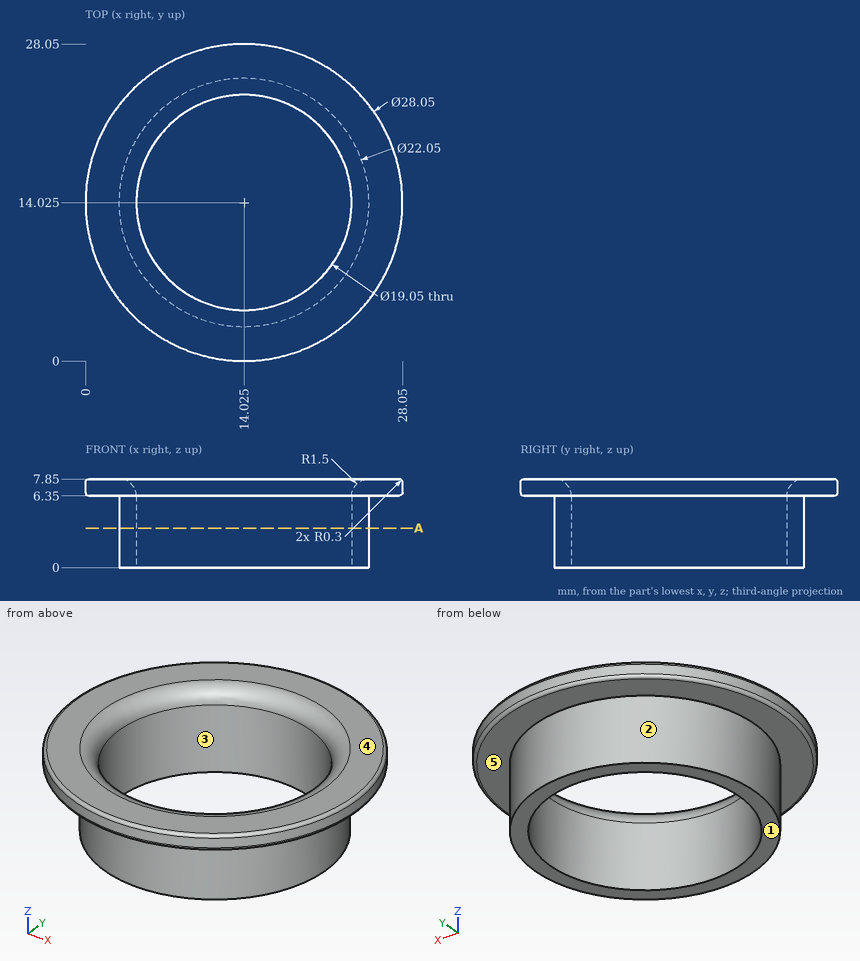
Could you check a few things on this drawing? It's one solid part, dimensions in mm from its lowest x, y, z. A direction names the side the tool comes from. Give positions to 0.01 mm unless a question says otherwise; leave off trailing zeros. Order: outer loops, then holes, each group sorted by start corner. A loop starts at its lowest first (then second) coordinate and runs counter-clockwise, first axis right, second up. Notation, with made-up numbers: M -16.75,-18 L -0.75,-18 A19 cw -0.75,14 Z; hole C -12.5,35 d10. An arc over 180 degrees is marked long. Use one line per item in the form item = value. Start each with the question number.
Item 1: Will these pins go through, and if not, where does the flat tip stop? pin 1 Ø1 at (y, z) = (12, 5.5) entering from -X; pin 2 Ø3 at (y, z) = (12, 4.5) entering from -X; pin 3 Ø2 at (x, z) = (12, 1.5) entering from -Y.
Item 2: If we section it at A-A (z = 3.5): Write out the boundary of the cut face in (x, y) (3 decimals), then the cut area to 3 significant figures.
Item 3: For the marked faces 4 and 5, which set-ups out of +Z, -Z, +X, -X, +Y, -Y let a thin tool reach every point of the face, with its end or its side?
Item 4: We'd pull the mould along X, two halves only. Please class the marked faces 1, 2 and 3: +X half, -X half, draft (parallel to the pull), parting line (faces both ways), or undercut.
Item 5: If I drill on line 1 along Z through (x, y) = (24.25, 19); line 2 along X through (y, z) = (20.5, 7.25); line 3 along Y through (x, z) = (11, 5), over which ranges is the centre line in solid material (lowest first)?
Outcome:
q1.pin_1 = 3.11
q1.pin_2 = 3.01
q1.pin_3 = 3.05
q2.outline = C 14.025,14.025 d22.05; hole C 14.025,14.025 d19.05
q2.area = 96.8 mm2
q3.face_4 = +Z, +X, -X, +Y, -Y
q3.face_5 = -Z
q4.face_1 = draft
q4.face_2 = parting line
q4.face_3 = undercut
q5.line_1 = 6.35 to 7.85
q5.line_2 = 1.58 to 6.64, 21.41 to 26.47
q5.line_3 = 3.42 to 4.99, 23.06 to 24.63
